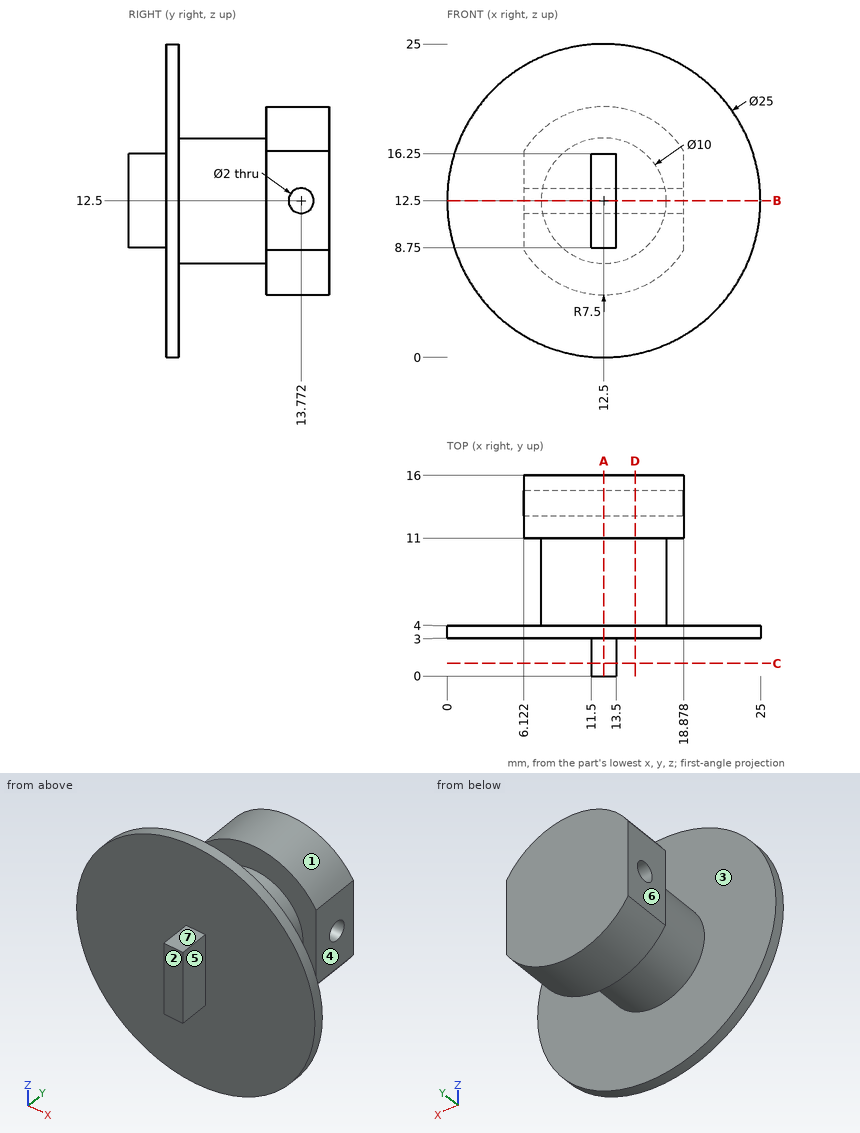
Part print with two shaded views. Sizes in mm from the minimum x, y, z corner. A direction names the side the tool comes from. Round coordinates to 2 decimals unless told otherwise and drop trailing zeros. Write each loop counter-clockwise with the first axis right and the second up, starting at its lowest first coordinate (ties: lowest second). Pieces come first, ordered by that corner, then holes. Notation, with made-up numbers: M 45,-8.5 L 89,-8.5 A17 ccw 89,-3.5 Z; hole C 15,73 d4. An arc over 180 degrees is marked long. Answer as CSV lines item,"result". Start each with the question number.
1) Which spindle directions (+Z, -Z, +X, -X, +Y, -Y) get a long thin tool onto all of the face, cutting with end or side? Do the marked faces 4, 5, 6 and 7. Say none if no direction does.
2) Band-saw the part on C-C (y = 1). List the corners of the cut face in (x, z), then the cut area to 3 significant figures.
3) Band-saw the part on B-B (z = 12.5). List the corners of the cut face in (x, y), then the cut area to 3 significant figures.
4) Drop flat-ended pins along their axis: pin 1 (2 mm diameter, centred on x = 5, y = 3, fed in from -Z); pin 2 (1.6 mm diameter, centred on x = 12, y = 2, fed in from -Z); pin 3 (12 mm diameter, centred on x = 7, z = 3.5, fed in from -Y). Give the stop position or say it passes through.
5) Band-saw the part on D-D (x = 15). List the corners of the cut face in (y, z).
6) Band-saw the part on A-A (x = 12.5). List the corners of the cut face in (y, z).
7) Drill centre lines: L1, parallel to Y at x = 7.25, z = 10.75; L2, parallel to Y at x = 8.5, z = 10; L3, parallel to Y at x = 3.75, z = 3.75. Where is each one in solid material? Low to high.
8) Mould opens along Y. For the marked faces 1, 2 and 3 say: +Y half, -Y half, draft (parallel to the pull), parting line (faces both ways), or undercut.
Worked out:
1,face 4,"+Z, -Z, +X, +Y"
1,face 5,"+Z, -Z, +X, -Y"
1,face 6,"+Z, -Z, -X, +Y"
1,face 7,"+Z, +X, -X, -Y"
2,outline,"M 11.5,8.75 L 13.5,8.75 L 13.5,16.25 L 11.5,16.25 Z"
2,area,"15.0 mm²"
3,outline,"M 0,3 L 11.5,3 L 11.5,0 L 13.5,0 L 13.5,3 L 25,3 L 25,4 L 17.5,4 L 17.5,11 L 18.88,11 L 18.88,12.77 L 6.12,12.77 L 6.12,11 L 7.5,11 L 7.5,4 L 0,4 Z; M 6.12,14.77 L 18.88,14.77 L 18.88,16 L 6.12,16 Z"
3,area,"139 mm²"
4,pin 1,"z = 1.82"
4,pin 2,"z = 8.75"
4,pin 3,"y = 3"
5,outline,"M 3,0.25 L 4,0.25 L 4,8.17 L 11,8.17 L 11,5.43 L 16,5.43 L 16,19.57 L 11,19.57 L 11,16.83 L 4,16.83 L 4,24.75 L 3,24.75 Z; hole C 13.77,12.5 d2"
6,outline,"M 0,8.75 L 3,8.75 L 3,0 L 4,0 L 4,7.5 L 11,7.5 L 11,5 L 16,5 L 16,20 L 11,20 L 11,17.5 L 4,17.5 L 4,25 L 3,25 L 3,16.25 L 0,16.25 Z; hole C 13.77,12.5 d2"
7,L1,"3 to 4, 11 to 16"
7,L2,"3 to 16"
7,L3,"3 to 4"
8,face 1,"draft"
8,face 2,"-Y half"
8,face 3,"undercut"
